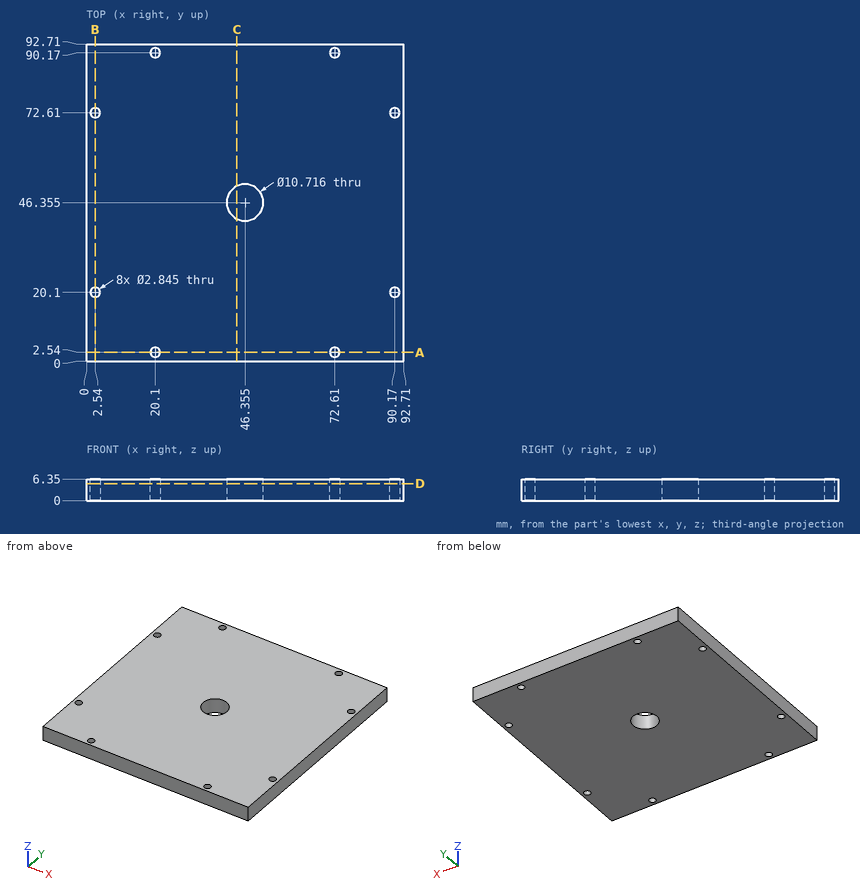
Here's the drawing with two shaded views (mm, measured from the low corner). I have some questions. Coordinates: 2 decimals unless noted, no trailing zeros. Write each loop counter-clockwise with the first axis right and the second up, starting at its lowest first coordinate (ties: lowest second). Pieces come first, ordered by that corner, then holes.
Item 1: If I drill on line 1 (Y direction, x = 2.54, z = 2); line 2 (X direction, y = 20.5, z = 4.75) (1 decimal); line 3 (Y direction, x = 73, z = 0.5), over which ranges is the centre line in solid material (lowest first)?
Item 2: I want a section at A-A on y = 2.54. Write out the boundary of the cut face in (x, z).
Item 3: Will this pin go through, and if not, where does the flat tip stop? pin 1 (2.5 mm diameter, centred on x = 72.61, y = 90.17, fed in from -Z).
Item 4: I want a section at C-C on x = 44. Write out the boundary of the cut face in (y, z).
Item 5: I want a section at D-D on z = 5. Count the separate pieces of the cut face and the enclosed holes in it, and give its area (3 significant figures).
Findings below:
1. line 1: y = 0 to 18.68, 21.52 to 71.19, 74.03 to 92.71
1. line 2: x = 0 to 1.2, 3.9 to 88.8, 91.5 to 92.7
1. line 3: y = 0 to 1.17, 3.91 to 88.8, 91.54 to 92.71
2. outline: (0, 0) - (18.68, 0) - (18.68, 6.35) - (0, 6.35) - close; (21.52, 0) - (71.19, 0) - (71.19, 6.35) - (21.52, 6.35) - close; (74.03, 0) - (92.71, 0) - (92.71, 6.35) - (74.03, 6.35) - close
3. pin 1: passes through
4. outline: (0, 0) - (41.54, 0) - (41.54, 6.35) - (0, 6.35) - close; (51.17, 0) - (92.71, 0) - (92.71, 6.35) - (51.17, 6.35) - close
5. separate pieces: 1
5. enclosed holes: 9
5. area: 8,450 mm2
